```python
from build123d import *

# Parameters (mm, degrees)
F0_R     = 32.5
F1_DEPTH = 4
F2_R     = 22.5
F3_DEPTH = 12.5
F4_R     = 19.5
F5_DEPTH = 30
F6_R     = 15.5
F7_DEPTH = 46.501
F8_R     = 2
F9_DEPTH = 4.001
F10_SIZE = 2
F11_SIZE = 1


with BuildPart() as f1:
    # F0 (on Top) → F1 (new body)
    with BuildSketch(Plane.XY):
        Circle(F0_R)
    extrude(amount=F1_DEPTH)

    # F2 (on face) → F3 (join)
    with BuildSketch(Plane.XY.offset(4)):
        Circle(F2_R)
    extrude(amount=F3_DEPTH)

    # F4 (on face) → F5 (join)
    with BuildSketch(Plane.XY.offset(16.5)):
        Circle(F4_R)
    extrude(amount=F5_DEPTH)

    # F6 (on face) → F7 (cut, through all)
    with BuildSketch(Plane.XY.offset(46.5)):
        Circle(F6_R)
    extrude(amount=-F7_DEPTH, mode=Mode.SUBTRACT)

    # F8 (on face) → F9 (cut, through all)
    with BuildSketch(Plane.XY.offset(4)):
        with Locations((0, 27.5)):
            Circle(F8_R)
        with Locations((27.5, 0)):
            Circle(F8_R)
        with Locations((0, -27.5)):
            Circle(F8_R)
        with Locations((-27.5, 0)):
            Circle(F8_R)
    extrude(amount=-F9_DEPTH, mode=Mode.SUBTRACT)

    # F10
    f10_edges = [f1.edges().sort_by_distance(p)[0] for p in [
        (-19.5, 0, 46.5),
    ]]
    chamfer(f10_edges, length=F10_SIZE)

    # F11
    f11_edges = [f1.edges().sort_by_distance(p)[0] for p in [
        (-22.5, 0, 16.5),
    ]]
    chamfer(f11_edges, length=F11_SIZE)


solid = f1.part
```
Build history of the part. All positions in model axes, mm. A direction names the side the tool comes from. Give positions to 0.01 mm unless a question says otherwise; leave off trailing zeros. Loops run counter-clockwise (first coordinate to the right, second up) from the corner with the lowest first, then second, coordinate; pieces in that order, holes last.
1) Probe line 1 along Y through (x, z) = (0, 2.65); line 2 along Y through (x, z) = (0, 27.5); line 3 along Z through (x, y) = (22.5, 23). List the from-to ranges inside material, lowest first.
Values follow:
line 1: y = -32.5 to -29.5, -25.5 to -15.5, 15.5 to 25.5, 29.5 to 32.5
line 2: y = -19.5 to -15.5, 15.5 to 19.5
line 3: z = 0 to 4
2) Band-saw the part on C-C on x = -27.5. List the corners of the cut face in (y, z), then the cut area to 3 significant figures.
Values follow:
outline: (-17.32, 0) - (-2, 0) - (-2, 4) - (-17.32, 4) - close; (2, 0) - (17.32, 0) - (17.32, 4) - (2, 4) - close
area: 123 mm2
3) Two-plate mould, pull along Y, no slides. Class faces 1 (the face through (-25.592, 0.601, 2.028)), 2 (the face through (16.811, 5.294, 46.375)), 3 (the face through (-7, -14, 46.5)), 4 (the face through (29.408, 0.601, 2.028)): released by +Y, released by -Y, zero draft, split by the parting line, or undercut.
Values follow:
face 1: undercut
face 2: split by the parting line
face 3: zero draft
face 4: undercut
4) 3-axis set-ups, long thin cutter, end or side, ignore diameter. For faces 5 (the face through (7, 22, 4)), 6 (the face through (-0.434, -29.452, 2.028)): which of +Z, -Z, +X, -X, +Y, -Y reach the whole face in a straight line?
Values follow:
face 5: +Z
face 6: +Z, -Z
5) Drop flat-ended pins along their axis: P1, Ø1.5, axis at x = -4, y = 18, coming from the +Z side; P2, Ø12, axis at x = 18, z = 34.5, coming from the +Y side; P3, Ø5, axis at x = 0, y = -27.5, coming from the -Z side; P4, Ø1.5, axis at y = -5.5, z = 41, coming from the -X side. Give the stop position or say it passes through.
Values follow:
P1: stops at z = 46.31
P2: stops at y = 15.37
P3: stops at z = 0
P4: stops at x = -18.91
6) Band-saw the part on B-B on z = 3. List the corners of the cut face in (x, y), then the cut area to 3 significant figures.
Values follow:
outline: circle Ø65 at (0, 0); hole circle Ø4 at (-27.5, 0); hole circle Ø31 at (0, 0); hole circle Ø4 at (0, -27.5); hole circle Ø4 at (0, 27.5); hole circle Ø4 at (27.5, 0)
area: 2,510 mm2
7) Band-saw the part on A-A on y = 0. List the corners of the cut face in (x, z).
Values follow:
outline: (-32.5, 0) - (-29.5, 0) - (-29.5, 4) - (-32.5, 4) - close; (-25.5, 0) - (-15.5, 0) - (-15.5, 46.5) - (-17.5, 46.5) - (-19.5, 44.5) - (-19.5, 16.5) - (-21.5, 16.5) - (-22.5, 15.5) - (-22.5, 4) - (-25.5, 4) - close; (15.5, 0) - (25.5, 0) - (25.5, 4) - (22.5, 4) - (22.5, 15.5) - (21.5, 16.5) - (19.5, 16.5) - (19.5, 44.5) - (17.5, 46.5) - (15.5, 46.5) - close; (29.5, 0) - (32.5, 0) - (32.5, 4) - (29.5, 4) - close
